```python
from build123d import *

# Parameters (mm, degrees)
F1_DEPTH = 3.5
F2_R     = 10.65
F3_DEPTH = 7


with BuildPart() as f1:
    # F0 (on Top) → F1 (new body, symmetric)
    with BuildSketch(Plane.XY):
        with BuildLine():
            ThreePointArc((11.2249721603, -5.5), (12.1770717335, -2.8229282665), (12.5, 0))
            ThreePointArc((12.5, 0), (8.8388347648, 8.8388347648), (0, 12.5))
            ThreePointArc((0, 12.5), (-10.6066017178, 6.6143782777), (-11.2249721603, -5.5))
            ThreePointArc((-11.2249721603, -5.5), (0, -12.5), (11.2249721603, -5.5))
        make_face()
        with BuildLine():
            ThreePointArc((0, 12.5), (8.8388347648, 8.8388347648), (12.5, 0))
            ThreePointArc((12.5, 0), (12.1770717335, -2.8229282665), (11.2249721603, -5.5))
            Line((11.2249721603, -5.5), (23.3493278133, 1.5))
            ThreePointArc((23.3493278133, 1.5), (33.9559295311, 20.6143782777), (12.124355653, 19.5))
            Line((12.124355653, 19.5), (0, 12.5))
        make_face()
        with BuildLine():
            ThreePointArc((-11.2249721603, -5.5), (-10.6066017178, 6.6143782777), (0, 12.5))
            Line((0, 12.5), (-12.124355653, 19.5))
            ThreePointArc((-12.124355653, 19.5), (-33.9559295311, 20.6143782777), (-23.3493278133, 1.5))
            Line((-23.3493278133, 1.5), (-11.2249721603, -5.5))
        make_face()
        with BuildLine():
            Line((11.2249721603, -19.5), (11.2249721603, -5.5))
            ThreePointArc((11.2249721603, -5.5), (0, -12.5), (-11.2249721603, -5.5))
            Line((-11.2249721603, -5.5), (-11.2249721603, -19.5))
            ThreePointArc((-11.2249721603, -19.5), (0, -37.5), (11.2249721603, -19.5))
        make_face()
    extrude(amount=F1_DEPTH, both=True)

    # F2 (on face) → F3 (cut, symmetric)
    with BuildSketch(Plane.XY.offset(3.5)):
        with Locations((-23.3493278133, 14)):
            Circle(F2_R)
        Circle(F2_R)
        with Locations((23.3493278133, 14)):
            Circle(F2_R)
        with Locations((0, -25)):
            Circle(F2_R)
    extrude(amount=F3_DEPTH, both=True, mode=Mode.SUBTRACT)


solid = f1.part
```
Design review of the part built by this model. Coordinates are the model's own, in mm. A direction names the side the tool comes from. Give positions to 0.01 mm unless a question says otherwise; leave off trailing zeros. Loops run counter-clockwise (first coordinate to the right, second up) from the corner with the lowest first, then second, coordinate; pieces in that order, holes last. Notation, with made-up numbers: M -14.5,38.5 L -7.5,38.5 A13 ccw -7.5,55.5 Z; hole C 29,69 d8. An arc over 180 degrees is marked long. Return JSON: item names as keys, results as strings. Group by question number.
Item 1: We need section B-B (z = -0.5). Give the boundary of the cut face in (x, y).
Item 2: Insertion check: pin 1 Ø1.5 at (x, z) = (5.5, -1.5) entering from -Y; pin 2 Ø17 at (x, y) = (23.35, 14) entering from +Z; pin 3 Ø1 at (y, z) = (-30, 2.5) entering from -X; pin 4 Ø2 at (x, z) = (-15.5, -2) entering from -Y. Each pin has a flat end and moves straight along its axis. Give the tip position at first contact, or say it passes through.
Item 3: Tool access review of faces 4 (the flat face through (11.225, -13, 0)), 5 (the cylindrical face through (34.148, 20.295, 0.049)), 6 (the flat face through (0, 11, -3.5)), 7 (the flat face through (-5.977, 15.951, 0.049)), 8 (the flat face through (-11.225, -12, 0)): name each direction out of +Z, -Z, +X, -X, +Y, -Y from which nothing blocks a thin tool from reaching the whole face with its end or side.
Item 4: We need section A-A (y = -25). Give the boundary of the cut face in (x, z).
Item 5: For probe 1 along Y at (x, z) = (0, 0.75); probe 2 along X at (y, z) = (5.5, -2); probe 3 along X at (y, z) = (14.5, -3), list the stretches that pass through material, from the lowest coordinate up.
Item 6: Mouldability with a two-part tool opening along Y and no side actions: class faces 1 (the cylindrical face through (-31.199, 21.198, 0.049)), 2 (the flat face through (6.15, 16.05, 0.05)), 3 (the cylindrical face through (-33.754, 20.927, 0.049)) as released by +Y, released by -Y, zero draft, split by the parting line, or undercut.
Item 7: We need section D-D (y = 14). Give the boundary of the cut face in (x, z), and give its area (3 significant figures).
Item 8: We need section C-C (x = -18). Give the boundary of the cut face in (y, z), and give its area (3 significant figures).
Output:
{
 "1": {"outline": "M -23.35,1.5 L -11.22,-5.5 L -11.22,-19.5 A12.5 ccw long 11.22,-19.5 L 11.22,-5.5 L 23.35,1.5 A12.5 ccw long 12.12,19.5 L 0,12.5 L -12.12,19.5 A12.5 ccw long Z; hole C -23.35,14 d21.3; hole C 0,-25 d21.3; hole C 0,0 d21.3; hole C 23.35,14 d21.3"},
 "2": {"pin 1": "stops at y = -36.56", "pin 2": "passes through", "pin 3": "stops at x = -11.66", "pin 4": "stops at y = -3.61"},
 "3": {"face 4": "+Z, -Z, +X", "face 5": "+Z, -Z", "face 6": "-Z, +X, -X, +Y, -Y", "face 7": "+Z, -Z, +Y", "face 8": "+Z, -Z, -X"},
 "4": {"outline": "M -12.5,-3.5 L -10.65,-3.5 L -10.65,3.5 L -12.5,3.5 Z; M 10.65,-3.5 L 12.5,-3.5 L 12.5,3.5 L 10.65,3.5 Z"},
 "5": {"probe 1": "y = -37.5 to -35.65, -14.35 to -10.65, 10.65 to 12.5", "probe 2": "x = -32.51 to -29.77, -16.93 to -9.12, 9.12 to 16.93, 29.77 to 32.51", "probe 3": "x = -35.84 to -33.99, -12.71 to -3.46, 3.46 to 12.71, 33.99 to 35.84"},
 "6": {"face 1": "undercut", "face 2": "released by +Y", "face 3": "split by the parting line"},
 "7": {"outline": "M -35.85,-3.5 L -34,-3.5 L -34,3.5 L -35.85,3.5 Z; M -12.7,-3.5 L -2.6,-3.5 L -2.6,3.5 L -12.7,3.5 Z; M 2.6,-3.5 L 12.7,-3.5 L 12.7,3.5 L 2.6,3.5 Z; M 34,-3.5 L 35.85,-3.5 L 35.85,3.5 L 34,3.5 Z", "area": "167 mm^2"},
 "8": {"outline": "M -1.59,-3.5 L 4.79,-3.5 L 4.79,3.5 L -1.59,3.5 Z; M 23.21,-3.5 L 25.3,-3.5 L 25.3,3.5 L 23.21,3.5 Z", "area": "59.3 mm^2"}
}
